```python
from build123d import *

# Parameters (mm, degrees)
SKETCH1_R               = 4.191
SKETCH1_R_2             = 5.55625
BOSS_EXTRUDE1_DEPTH     = 33.02
CUT_EXTRUDE1_DEPTH      = 56.118
SKETCH3_W               = 26.483565884
SKETCH3_H               = 26.924
CUT_EXTRUDE2_DEPTH      = 11.12825
CUT_EXTRUDE2_DEPTH_BACK = 82.28
BOSS_EXTRUDE2_DEPTH     = 5.08


with BuildPart() as part:
    # Sketch1 → Boss-Extrude1 (new body)
    with BuildSketch(Plane(origin=(0, 0, 0), x_dir=(1, 0, 0), z_dir=(0, 1, 0))):
        with BuildLine():
            ThreePointArc((-27.559, -34.820535754), (-23.929058682, -42.090058682), (-16.659535754, -45.72))
            Line((-16.659535754, -45.72), (-13.058464246, -45.72))
            ThreePointArc((-13.058464246, -45.72), (-5.472288324, -41.761943314), (-2.063174534, -33.91374473))
            ThreePointArc((-2.063174534, -33.91374473), (-1.931764874, -32.906728948), (-1.680693889, -31.922700165))
            Line((-1.680693889, -31.922700165), (5.577256486, -9.252591406))
            Line((5.577256486, -9.252591406), (15.95594723, 23.165107224))
            ThreePointArc((15.95594723, 23.165107224), (17.206676654, 25.810946447), (19.103326913, 28.039736946))
            ThreePointArc((19.103326913, 28.039736946), (21.273883819, 30.828033828), (22.3544782, 34.19229193))
            ThreePointArc((22.3544782, 34.19229193), (22.881358513, 35.169970415), (23.921231105, 35.56))
            Line((23.921231105, 35.56), (27.559, 35.56))
            Line((27.559, 35.56), (27.559, 43.286638959))
            ThreePointArc((27.559, 43.286638959), (26.855584412, 44.984834412), (25.157388959, 45.68825))
            Line((25.157388959, 45.68825), (12.319, 45.68825))
            ThreePointArc((12.319, 45.68825), (6.28241864, 43.692719935), (2.624566002, 38.492472937))
            ThreePointArc((2.624566002, 38.492472937), (1.133892546, 36.373232242), (-1.326176925, 35.56))
            Line((-1.326176925, 35.56), (-26.38140718, 35.56))
            ThreePointArc((-26.38140718, 35.56), (-27.214091048, 35.215091048), (-27.559, 34.38240718))
            Line((-27.559, 34.38240718), (-27.559, -31.219464246))
            Line((-27.559, -31.219464246), (-27.559, -34.820535754))
        make_face()
        with Locations((-14.859, -33.02)):
            Circle(SKETCH1_R, mode=Mode.SUBTRACT)
        with Locations((12.319, 35.56)):
            Circle(SKETCH1_R_2, mode=Mode.SUBTRACT)
    extrude(amount=BOSS_EXTRUDE1_DEPTH)

    # Sketch2 → Cut-Extrude1 (cut, through all)
    with BuildSketch(Plane.ZY.offset(27.559)):
        Polygon((-31.33440718, 29.972), (42.672, 29.972), (45.72, 29.972), (45.72, 3.048), (42.672, 3.048), (-31.33440718, 3.048), align=None)
    extrude(amount=-CUT_EXTRUDE1_DEPTH, mode=Mode.SUBTRACT)

    # Sketch3 → Cut-Extrude2 (cut, two sides)
    with BuildSketch(Plane(origin=(0, 0, -35.56), x_dir=(-1, 0, 0), z_dir=(0, 0, -1))) as cut_extrude2_sk:
        with Locations((-11.915606017, 16.51)):
            Rectangle(SKETCH3_W, SKETCH3_H)
    extrude(amount=CUT_EXTRUDE2_DEPTH, mode=Mode.SUBTRACT)
    extrude(cut_extrude2_sk.sketch, amount=-CUT_EXTRUDE2_DEPTH_BACK, mode=Mode.SUBTRACT)

    # Sketch4 → Boss-Extrude2 (add)
    with BuildSketch(Plane(origin=(0, 33.02, 0), x_dir=(1, 0, 0), z_dir=(0, 1, 0))):
        with BuildLine():
            Line((21.209, 45.68825), (21.209, 35.56))
            Line((21.209, 35.56), (27.559, 35.56))
            Line((27.559, 35.56), (27.559, 43.286638959))
            ThreePointArc((27.559, 43.286638959), (26.855584412, 44.984834412), (25.157388959, 45.68825))
            Line((25.157388959, 45.68825), (21.209, 45.68825))
        make_face()
    boss_extrude2 = extrude(amount=BOSS_EXTRUDE2_DEPTH)

    # Mirror1: Boss-Extrude2 across plane
    add(boss_extrude2.mirror(Plane.ZX.offset(16.51)))


solid = part.part
```
Can you work these out from the model? Positions are in its coordinate system, mm. A direction names the side the tool comes from. Round coordinates to 2 decimals unless told otherwise and drop trailing zeros. Loops run counter-clockwise (first coordinate to the right, second up) from the corner with the lowest first, then second, coordinate; pieces in that order, holes last. Notation, with made-up numbers: (-22.75, -1) -> (19.25, -1) arc R5 ccw to (19.25, 6) -> close; hole circle Ø3 at (7, -15.75). An arc over 180 degrees is marked (long way). One line per item, written item: value. Start each with the question number.
1. If we mould it in two halves opening along Z, with no side actions, what happens to faces 1 (the flat face through (25.157, 16, -41)), 2 (the cylindrical face through (6.36, 1.5, -43.75)), 3 (the cylindrical face through (-10.86, 31.47, 31.76)), 4 (the cylindrical face through (17.2, 31.5, -25.8))? For each: pulls with the +Z half, pulls with the -Z half, needs draft (parallel to the pull), parting line crosses it, or undercut.
2. If we section it at D-D, the plane x = -22: Write out the boundary of the cut face in (y, z).
3. For pin 1 (8 mm diameter, centred on y = 13.5, z = -28, fed in from -X); pin 2 (5.5 mm diameter, centred on y = 35.5, z = -40.5, fed in from -X); pin 3 (15.5 mm diameter, centred on x = 0, z = -3.5, fed in from -Y); pin 4 (4 mm diameter, centred on x = -7, y = 24.5, fed in from +Z), each with a flat end and sliding along its axis, tell me the tip position at first contact or that it passes through.
4. If we section it at A-A, the plane z = -7: Write out the boundary of the cut face in (x, y).
5. If we section it at B-B, the plane x = 10: Write out the boundary of the cut face in (y, z), then the cut area to 3 significant figures.
6. For faces 5 (the cylindrical face through (11.6, 1.5, -41.07)), 6 (the flat face through (-15, 16, -31.334)), 7 (the flat face through (-1.326, 16, -33)), which set-ups out of +Z, -Z, +X, -X, +Y, -Y let a thin tool reach every point of the face, with its end or its side?
7. If we section it at C-C, the plane y = 26.5: Write out the boundary of the cut face in (x, z).
8. If I drill on probe 1 along Y at (x, z) = (-1, -18.5); probe 2 along Z at (x, y) = (-5, 13.5); probe 3 along Z at (x, y) = (-17, 31), over which ranges is the centre line in solid material (lowest first)?
Calculated:
1. face 1: needs draft
1. face 2: pulls with the -Z half
1. face 3: undercut
1. face 4: pulls with the +Z half
2. outline: (0, -35.56) -> (33.02, -35.56) -> (33.02, 43.68) -> (29.97, 43.68) -> (29.97, -31.33) -> (3.05, -31.33) -> (3.05, 43.68) -> (0, 43.68) -> close
3. pin 1: stops at x = -27.56
3. pin 2: stops at x = 2.91
3. pin 3: stops at y = 0
3. pin 4: stops at z = -31.33
4. outline: (-27.56, 0) -> (10.78, 0) -> (10.78, 3.05) -> (-27.56, 3.05) -> close; (-27.56, 29.97) -> (10.78, 29.97) -> (10.78, 33.02) -> (-27.56, 33.02) -> close
5. outline: (0, -45.42) -> (3.05, -45.42) -> (3.05, -40.61) -> (0, -40.61) -> close; (0, -30.51) -> (3.05, -30.51) -> (3.05, -4.56) -> (0, -4.56) -> close; (29.97, -45.42) -> (33.02, -45.42) -> (33.02, -40.61) -> (29.97, -40.61) -> close; (29.97, -30.51) -> (33.02, -30.51) -> (33.02, -4.56) -> (29.97, -4.56) -> close
5. area: 188 mm²
6. face 5: +Y, -Y
6. face 6: +Z, +X, -X
6. face 7: +Z, -Z, +X
7. outline: (-27.56, -34.38) arc R1.18 ccw to (-26.38, -35.56) -> (-1.33, -35.56) -> (-1.33, -31.33) -> (-27.56, -31.33) -> close; (25.16, -45.69) arc R2.4 ccw to (27.56, -43.29) -> (27.56, -35.56) -> (25.16, -35.56) -> close
8. probe 1: y = 0 to 3.05, 29.97 to 33.02
8. probe 2: z = -35.56 to -31.33
8. probe 3: z = -35.56 to 29.42, 36.62 to 45.67
